Check sheet for the modelled part. Datum: model origin and axes. Units: mm. Face numbers are marked on the shaded views. A direction names the side the tool comes from. Give positions to 0.01 mm unless a question says otherwise; leave off trailing zeros. Loops run counter-clockwise (first coordinate to the right, second up) from the corner with the lowest first, then second, coordinate; pieces in that order, holes last. Notation, with made-up numbers: M 47,-38 L 55,-38 A16 cw 55,-14 Z; hole C 7,-18.5 d10. An arc over 180 degrees is marked long. Use one line per item in the form item = value.
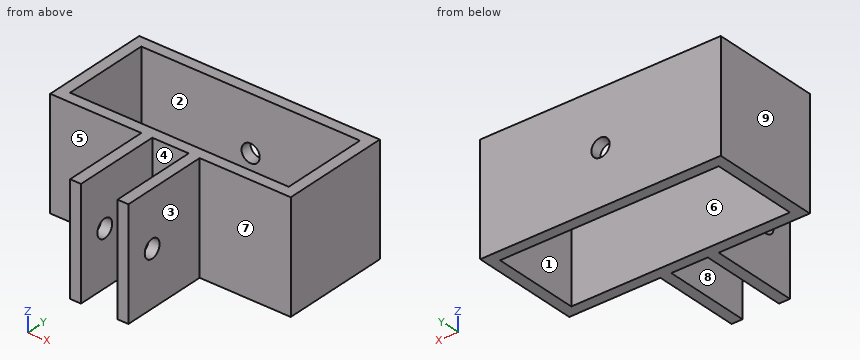
from build123d import *

# Parameters (mm, degrees)
SKETCH1_W           = 66
SKETCH1_H           = 30
BOSS_EXTRUDE1_DEPTH = 30
SKETCH2_W           = 30
SKETCH2_H           = 24
CUT_EXTRUDE1_DEPTH  = 54.749418602
SKETCH3_R           = 2.5
CUT_EXTRUDE2_DEPTH  = 10
SKETCH4_W           = 16
SKETCH4_H           = 30
BOSS_EXTRUDE2_DEPTH = 24
SKETCH5_W           = 10
SKETCH5_H           = 24
CUT_EXTRUDE3_DEPTH  = 54.749418602
SKETCH6_R           = 2.5
CUT_EXTRUDE4_DEPTH  = 24


with BuildPart() as part:
    # Sketch1 → Boss-Extrude1 (new body)
    with BuildSketch(Plane(origin=(0, 0, 0), x_dir=(1, 0, 0), z_dir=(0, 1, 0))):
        Rectangle(SKETCH1_W, SKETCH1_H)
    extrude(amount=BOSS_EXTRUDE1_DEPTH)

    # Sketch2 → Cut-Extrude1 (cut, through all)
    with BuildSketch(Plane.XY.offset(15)):
        with Locations((15, 15)):
            Rectangle(SKETCH2_W, SKETCH2_H)
        with Locations((-15, 15)):
            Rectangle(SKETCH2_W, SKETCH2_H)
    extrude(amount=-CUT_EXTRUDE1_DEPTH, mode=Mode.SUBTRACT)

    # Sketch3 → Cut-Extrude2 (cut)
    with BuildSketch(Plane(origin=(0, 30, 0), x_dir=(1, 0, 0), z_dir=(0, 1, 0))):
        with Locations(Location((0, 0, 0), (0, 0, 270))):
            Circle(SKETCH3_R)
    extrude(amount=-CUT_EXTRUDE2_DEPTH, mode=Mode.SUBTRACT)

    # Sketch4 → Boss-Extrude2 (add)
    with BuildSketch(Plane.XZ):
        Rectangle(SKETCH4_W, SKETCH4_H)
    extrude(amount=BOSS_EXTRUDE2_DEPTH)

    # Sketch5 → Cut-Extrude3 (cut, through all)
    with BuildSketch(Plane.XY.offset(15)):
        with Locations((0, -12)):
            Rectangle(SKETCH5_W, SKETCH5_H)
    extrude(amount=-CUT_EXTRUDE3_DEPTH, mode=Mode.SUBTRACT)

    # Sketch6 → Cut-Extrude4 (cut)
    with BuildSketch(Plane(origin=(8, 0, 0), x_dir=(0, 0, -1), z_dir=(1, 0, 0))):
        with Locations((0, -16)):
            Circle(SKETCH6_R)
    extrude(amount=-CUT_EXTRUDE4_DEPTH, mode=Mode.SUBTRACT)


solid = part.part
1) Set-up check for the marked faces 5, 6, 7, 8 and 9: record each of +Z, -Z, +X, -X, +Y, -Y from which the full face is reachable in a straight line by a thin tool's end or side.
Evaluation:
face_5 = +Z, -Z, -X, -Y
face_6 = +Z, -Z
face_7 = +Z, -Z, +X, -Y
face_8 = +Z, -Z, -Y
face_9 = +Z, -Z, -X, +Y, -Y
2) Depth check by flat-ended pin: pin 1 Ø3 at (x, z) = (18.5, 8.5) entering from -Y; pin 2 Ø1.5 at (y, z) = (-4, -7) entering from -X; pin 3 Ø12 at (y, z) = (-10.5, 4.5) entering from +X; pin 4 Ø4.5 at (y, z) = (-16, 0) entering from +X. Enter the tip coordinate at first touch or a pass-through.
Evaluation:
pin_1 = 0
pin_2 = -8
pin_3 = 8
pin_4 = through
3) Section check A-A (y = -4). Record the cut outline in (x, z), then the cut area to 3 significant figures.
Evaluation:
outline = M -8,-15 L -5,-15 L -5,15 L -8,15 Z; M 5,-15 L 8,-15 L 8,15 L 5,15 Z
area = 180 mm^2
4) Scan lines: line 1 (Y direction, x = -6.45, z = 0); line 2 (Y direction, x = 21, z = 12.5); line 3 (X direction, y = 11, z = 8). Record each from-to range of solid material in increasing order.
Evaluation:
line_1 = -24 to -18.5, -13.5 to 3, 27 to 30
line_2 = 0 to 3, 27 to 30
line_3 = -33 to -30, 30 to 33
5) Release check for a two-part mould opening along Y. For the marked faces 1, 2, 3 and 4 record: pulls with the +Y half, pulls with the -Y half, needs draft (parallel to the pull), parting line crosses it, or undercut.
Evaluation:
face_1 = undercut
face_2 = undercut
face_3 = needs draft
face_4 = pulls with the -Y half
6) Section check C-C (x = 12). Record the cut outline in (y, z), then the cut area to 3 significant figures.
Evaluation:
outline = M 0,-15 L 3,-15 L 3,15 L 0,15 Z; M 27,-15 L 30,-15 L 30,15 L 27,15 Z
area = 180 mm^2
7) Section check B-B (z = 0). Record the cut outline in (x, y).
Evaluation:
outline = M -33,0 L -8,0 L -8,-13.5 L -5,-13.5 L -5,0 L 5,0 L 5,-13.5 L 8,-13.5 L 8,0 L 33,0 L 33,30 L 2.5,30 L 2.5,27 L 30,27 L 30,3 L -30,3 L -30,27 L -2.5,27 L -2.5,30 L -33,30 Z; M -8,-24 L -5,-24 L -5,-18.5 L -8,-18.5 Z; M 5,-24 L 8,-24 L 8,-18.5 L 5,-18.5 Z
8) Section check D-D (z = 7.5). Record the cut outline in (x, y), then the cut area to 3 significant figures.
Evaluation:
outline = M -33,0 L -8,0 L -8,-24 L -5,-24 L -5,0 L 5,0 L 5,-24 L 8,-24 L 8,0 L 33,0 L 33,30 L -33,30 Z; hole M -30,3 L 30,3 L 30,27 L -30,27 Z
area = 684 mm^2
